The listing builds one solid part. Answer for the finished solid, in the listing's coordinates (mm). A direction names the side the tool comes from. Coordinates: 2 decimals unless noted, no trailing zeros. Order: outer loops, then holes, each group sorted by start corner. A loop starts at its lowest first (then second) coordinate and runs counter-clockwise, first axis right, second up.
```python
from build123d import *

# Parameters (mm, degrees)
PAD_DEPTH       = 2.5
SKETCH001_W     = 19.2
SKETCH001_H     = 30
POCKET_DEPTH    = 3.3
SKETCH002_W     = 3
SKETCH002_H     = 10
PAD001_DEPTH    = 14
POCKET004_DEPTH = 5
SKETCH005_R     = 1
POCKET005_DEPTH = 26
CHAMFER_SIZE    = 3
FILLET_R        = 1
FILLET001_R     = 1
FILLET002_R     = 1
FILLET003_R     = 3
SKETCH007_R     = 8.5
POCKET006_DEPTH = 5
FILLET004_R     = 4.5


with BuildPart() as part:
    # Sketch → Pad (new body, symmetric)
    with BuildSketch(Plane.XY):
        with BuildLine():
            Line((-20, 20), (20, 20))
            ThreePointArc((30, 10), (27.071068, 17.071068), (20, 20))
            Line((30, 10), (30, -10))
            ThreePointArc((20, -20), (27.071068, -17.071068), (30, -10))
            Line((20, -20), (-20, -20))
            ThreePointArc((-30, -10), (-27.071068, -17.071068), (-20, -20))
            Line((-30, -10), (-30, 10))
            ThreePointArc((-20, 20), (-27.071068, 17.071068), (-30, 10))
        make_face()
    extrude(amount=PAD_DEPTH, both=True)

    # Sketch001 → Pocket (cut)
    with BuildSketch(Plane(origin=(0, 0, -2.5), x_dir=(1, 0, 0), z_dir=(0, 0, -1))):
        Rectangle(SKETCH001_W, SKETCH001_H)
    extrude(amount=-POCKET_DEPTH, mode=Mode.SUBTRACT)

    # Sketch002 (on Face4 of Pocket) → Pad001 (join)
    with BuildSketch(Plane(origin=(0, 0, -2.5), x_dir=(1, 0, 0), z_dir=(0, 0, -1))):
        with Locations((11.1, -3)):
            Rectangle(SKETCH002_W, SKETCH002_H)
        with Locations((-11.1, -3)):
            Rectangle(SKETCH002_W, SKETCH002_H)
    extrude(amount=PAD001_DEPTH)

    # Sketch004 → Pocket004 (cut)
    with BuildSketch(Plane.XY.offset(2.5)):
        with BuildLine():
            ThreePointArc((-21.75, 3), (-24, 5.25), (-26.25, 3))
            Line((-26.25, 3), (-26.25, -3))
            ThreePointArc((-26.25, -3), (-24, -5.25), (-21.75, -3))
            Line((-21.75, -3), (-21.75, 3))
        make_face()
        with BuildLine():
            ThreePointArc((26.25, 3), (24, 5.25), (21.75, 3))
            Line((21.75, 3), (21.75, -3))
            ThreePointArc((21.75, -3), (24, -5.25), (26.25, -3))
            Line((26.25, -3), (26.25, 3))
        make_face()
    extrude(amount=-POCKET004_DEPTH, mode=Mode.SUBTRACT)

    # Sketch005 (on Face21 of Pocket004) → Pocket005 (cut)
    with BuildSketch(Plane.YZ.offset(12.6)):
        with Locations((3, -9.5)):
            Circle(SKETCH005_R)
    extrude(amount=-POCKET005_DEPTH, mode=Mode.SUBTRACT)

    # Chamfer
    chamfer_edges = [part.edges().sort_by_distance(p)[0] for p in [
        (0, -15, -2.5),
        (0, 15, -2.5),
    ]]
    chamfer(chamfer_edges, length=CHAMFER_SIZE)

    # Fillet
    fillet_edges = [part.edges().sort_by_distance(p)[0] for p in [
        (-12.6, 3, -2.5),
    ]]
    fillet(fillet_edges, radius=FILLET_R)

    # Fillet001
    fillet001_edges = [part.edges().sort_by_distance(p)[0] for p in [
        (12.6, 3, -2.5),
    ]]
    fillet(fillet001_edges, radius=FILLET001_R)

    # Fillet002
    fillet002_edges = [part.edges().sort_by_distance(p)[0] for p in [
        (11.1, -2, -2.5),
        (-11.1, -2, -2.5),
        (11.1, 8, -2.5),
        (-11.1, 8, -2.5),
    ]]
    fillet(fillet002_edges, radius=FILLET002_R)

    # Fillet003
    fillet003_edges = [part.edges().sort_by_distance(p)[0] for p in [
        (0, 20, 2.5),
        (27.071068, 17.071068, 2.5),
        (30, 0, 2.5),
        (27.071068, -17.071068, 2.5),
        (0, -20, 2.5),
        (-27.071068, -17.071068, 2.5),
        (-30, 0, 2.5),
        (-27.071068, 17.071068, 2.5),
    ]]
    fillet(fillet003_edges, radius=FILLET003_R)

    # Sketch007 (on Face20 of Fillet003) → Pocket006 (cut)
    with BuildSketch(Plane(origin=(0, 20, 0), x_dir=(-1, 0, 0), z_dir=(0, 1, 0))):
        with Locations((0, -9.54)):
            Circle(SKETCH007_R)
    extrude(amount=-POCKET006_DEPTH, mode=Mode.SUBTRACT)

    # Fillet004
    fillet004_edges = [part.edges().sort_by_distance(p)[0] for p in [
        (-11.1, 8, -16.5),
        (-11.1, -2, -16.5),
        (11.1, -2, -16.5),
        (11.1, 8, -16.5),
    ]]
    fillet(fillet004_edges, radius=FILLET004_R)


solid = part.part
```
1) A cutting plane is placed at A-A, the plane z = -9.5. Write down the section's boundary in (x, y).
2) Each of these flat-tipped pins is pushed along its axis until it touches: P1, Ø1.2, axis at y = 3, z = -9.5, coming from the -X side; P2, Ø5, axis at x = -21, y = -5.5, coming from the -Z side; P3, Ø5, axis at y = 0.5, z = -10, coming from the +X side; P4, Ø2.5, axis at y = 3, z = -9.5, coming from the -X side. Where does it stop, or does it pass through?
3) A cutting plane is placed at C-C, the plane z = -6. Write down the section's boundary in (x, y), plus the area to 3 significant figures.
4) The mould has two halves that part along Y. Classify faces 1 (the cylindrical face through (0.28, 19.1, 1.64)), 2 (the cylindrical face through (-27.15, -16.99, -1.49)), 3 (the flat face through (9.6, 0, -6)): released by +Y, released by -Y, zero draft, split by the parting line, or undercut.
5) A cutting plane is placed at D-D, the plane y = -9. Write down the section's boundary in (x, z).
6) Straight lines are drawn through the part: probe 1 along Z at (x, y) = (-10, 3); probe 2 along X at (y, z) = (-0.5, -10.25); probe 3 along Z at (x, y) = (18.5, -7). For each, find the intervals that lie inside material, in ascending order.
7) For faces 4 (the flat face through (-30, 0, -1)), 5 (the flat face through (-11, -2, -8)), 6 (the flat face through (-21.75, 0, 0)), 7 (the cylindrical face through (-0.07, 18.6, -1.04)), 8 (the flat face through (-9.6, 0, -6)), determine the directions among +Z, -Z, +X, -X, +Y, -Y from which every point of the face is accessible in a straight line to the end or side of a thin tool.
8) A cutting plane is placed at B-B, the plane x = 11. Write down the section's boundary in (y, z), plus the area to 3 significant figures.
Working result:
1. outline: (-12.6, -2) - (-9.6, -2) - (-9.6, 2) - (-12.6, 2) - close; (-12.6, 4) - (-9.6, 4) - (-9.6, 8) - (-12.6, 8) - close; (9.6, -2) - (12.6, -2) - (12.6, 2) - (9.6, 2) - close; (9.6, 4) - (12.6, 4) - (12.6, 8) - (9.6, 8) - close
2. P1: passes through
2. P2: stops at z = -2.5
2. P3: stops at x = 12.6
2. P4: stops at x = -12.6
3. outline: (-12.6, -2) - (-9.6, -2) - (-9.6, 8) - (-12.6, 8) - close; (9.6, -2) - (12.6, -2) - (12.6, 8) - (9.6, 8) - close
3. area: 60.0 mm2
4. face 1: released by +Y
4. face 2: released by -Y
4. face 3: undercut
5. outline: (-30, -2.5) - (-9.6, -2.5) - (-9.6, 0.8) - (9.6, 0.8) - (9.6, -2.5) - (30, -2.5) - (30, -0.5) arc R3 ccw to (27, 2.5) - (-27, 2.5) arc R3 ccw to (-30, -0.5) - close
6. probe 1: z = -16.5 to -10.5, -8.5 to 2.5
6. probe 2: x = -12.6 to -9.6, 9.6 to 12.6
6. probe 3: z = -2.5 to 2.5
7. face 4: +Z, -Z, -X, +Y, -Y
7. face 5: -Z, +X, -X, -Y
7. face 6: +Z, -Z
7. face 7: -Z, +Y
7. face 8: -Z
8. outline: (-20, -2.5) - (-3, -2.5) arc R1 cw to (-2, -3.5) - (-2, -12) arc R4.5 ccw to (2.5, -16.5) - (3.5, -16.5) arc R4.5 ccw to (8, -12) - (8, -3.5) arc R1 cw to (9, -2.5) - (20, -2.5) - (20, -0.5) arc R3 ccw to (17, 2.5) - (-17, 2.5) arc R3 ccw to (-20, -0.5) - close; hole circle Ø2 at (3, -9.5)
8. area: 325 mm2
